For this review, take the finished solid that the model builds, in its own axes (mm). A direction names the side the tool comes from. Round coordinates to 2 decimals unless told otherwise and drop trailing zeros. Order: outer loops, then holes, each group sorted by start corner. A loop starts at its lowest first (then second) coordinate and runs counter-clockwise, first axis right, second up. Notation, with made-up numbers: M 50,37.25 L 101,37.25 A16 ccw 101,51.25 Z; hole C -9,41 d1. An arc over 180 degrees is marked long. Answer as a JSON object with one key per item and string values.
from build123d import *

# Parameters (mm, degrees)
SKETCH1_R           = 18
BOSS_EXTRUDE1_DEPTH = 6
SKETCH2_W           = 7.5
SKETCH2_H           = 21
CUT_EXTRUDE1_DEPTH  = 2


with BuildPart() as part:
    # Sketch1 → Boss-Extrude1 (new body)
    with BuildSketch(Plane(origin=(0, 0, 0), x_dir=(1, 0, 0), z_dir=(0, 1, 0))):
        with BuildLine():
            Line((-21.73544452, 25.635731314), (-12, 0))
            ThreePointArc((-12, 0), (0, -12), (12, 0))
            Line((12, 0), (21.73544452, 25.635731314))
            ThreePointArc((21.73544452, 25.635731314), (0, 57.14), (-21.73544452, 25.635731314))
        make_face()
        with Locations(Location((0, 33.89, 0), (0, 0, 270))):
            Circle(SKETCH1_R, mode=Mode.SUBTRACT)
    extrude(amount=BOSS_EXTRUDE1_DEPTH)

    # Sketch2 → Cut-Extrude1 (cut)
    with BuildSketch(Plane(origin=(0, 6, 0), x_dir=(1, 0, 0), z_dir=(0, 1, 0))):
        with Locations((0, 6.5)):
            Rectangle(SKETCH2_W, SKETCH2_H)
    extrude(amount=-CUT_EXTRUDE1_DEPTH, mode=Mode.SUBTRACT)


solid = part.part
1) Add section D-D on y = 1.75. State the section outline as (x, z) points, and give its area (3 significant figures).
Geometry check:
{"outline": "M -21.74,-25.64 A23.25 ccw long 21.74,-25.64 L 12,0 A12 ccw -12,0 Z; hole C 0,-33.89 d36", "area": "1,300 mm²"}
2) For L1, parallel to X at y = 2.85, z = -33.89; L2, parallel to Z at x = -0.5, y = 3.6; L3, parallel to X at y = 4.55, z = -26, list the stretches that pass through material, from the lowest coordinate up.
Geometry check:
{"L1": "x = -23.25 to -18, 18 to 23.25", "L2": "z = -57.13 to -51.88, -15.9 to 11.99", "L3": "x = -21.87 to -16.18, 16.18 to 21.87"}
3) Mouldability with a two-part tool opening along X and no side actions: class faces 3 (the flat face through (5, 6, -15)), 4 (the cylindrical face through (0.791, 2.958, -51.873)), 5 (the cylindrical face through (0.63, 2.96, -57.13)) as +X half, -X half, draft (parallel to the pull), parting line (faces both ways), or undercut.
Geometry check:
{"face 3": "draft", "face 4": "undercut", "face 5": "parting line"}
4) Insertion check: P1, Ø3, axis at y = 1.5, z = -26, coming from the -X side; P2, Ø1.5, axis at y = 4.5, z = -38.5, coming from the +X side; P3, Ø2, axis at y = 5.5, z = -3, coming from the +X side; P4, Ø21.5, axis at x = 0, z = -33.89, coming from the +Y side. Each pin has a flat end and moves straight along its axis. Give the tip position at first contact, or say it passes through.
Geometry check:
{"P1": "stops at x = -22.35", "P2": "stops at x = 22.93", "P3": "stops at x = 13.52", "P4": "passes through"}
5) Add section B-B on y = 4.8. State the section outline as (x, z) points.
Geometry check:
{"outline": "M -21.74,-25.64 A23.25 ccw long 21.74,-25.64 L 12,0 A12 ccw -12,0 Z; hole M -3.75,-16.28 A18 ccw long 3.75,-16.28 L 3.75,4 L -3.75,4 Z"}
6) Add section A-A on x = 0. State the section outline as (y, z) points, and give its area (3 significant figures).
Geometry check:
{"outline": "M 0,-57.14 L 6,-57.14 L 6,-51.89 L 0,-51.89 Z; M 0,-15.89 L 4,-15.89 L 4,4 L 6,4 L 6,12 L 0,12 Z", "area": "159 mm²"}
7) Machinability: for faces 1 (the flat face through (0, 4, -6)), 2 (the flat face through (16.8, 2.96, -12.64)), which of the approach directions +Z, -Z, +X, -X, +Y, -Y give a long, thin tool a straight path to every point of the face, cutting with its end or side? Answer none if there is none.
Geometry check:
{"face 1": "+Y", "face 2": "+Z, +X, +Y, -Y"}
8) Add section C-C on z = -41. State the section outline as (x, y) points, and give its area (3 significant figures).
Geometry check:
{"outline": "M -22.14,0 L -16.54,0 L -16.54,6 L -22.14,6 Z; M 16.54,0 L 22.14,0 L 22.14,6 L 16.54,6 Z", "area": "67.2 mm²"}
